Geometry check sheet. Reference: the model listing, model coordinates, mm. A direction names the side the tool comes from. Round coordinates to 2 decimals unless told otherwise and drop trailing zeros. Write each loop counter-clockwise with the first axis right and the second up, starting at its lowest first coordinate (ties: lowest second). Pieces come first, ordered by that corner, then holes.
Item 1: Cross-section at B-B (z = -0.2). State how many separate pieces and enclosed holes the cut face has, then the cut area to 3 significant figures.
Item 2: Cross-section at A-A (x = 70). Enter the section's corners in (y, z).
Item 3: Scan lines: probe 1 along Y at (x, z) = (0, -0.45); probe 2 along X at (y, z) = (0, -0.6); probe 3 along X at (y, z) = (-9.5, -0.05). Record each from-to range of solid material in increasing order.
Item 4: Depth check by flat-ended pin: P1, Ø3, axis at x = 77, y = -9.5, coming from the -Z side. Enter the tip coordinate at first touch or a pass-through.
Item 5: Access from +Z, -Z, +X, -X, +Y, -Y to the whole of each face (thin tool, end or side, straight path). Record for faces 1 (the face through (0, 7, -1.2)), 2 (the face through (79.1, -11.64, 0.02)), 3 (the face through (74, 0, 0)).
from build123d import *

# Parameters (mm, degrees)
SKETCH1_W                                            = 160
SKETCH1_H                                            = 25
BOSS_EXTRUDE1_DEPTH                                  = 1.5
SKETCH2_W                                            = 148
SKETCH2_H                                            = 13
CUT_EXTRUDE1_DEPTH                                   = 82.026230321
FILLET1_R                                            = 2
FILLET2_R                                            = 3
CSK_FOR_M2_SLOTTED_RAISED_CTSK_HEAD_SCRE_D           = 2.2
CSK_FOR_M2_SLOTTED_RAISED_CTSK_HEAD_SCRE_CSINK_D     = 4.5
CSK_FOR_M2_SLOTTED_RAISED_CTSK_HEAD_SCRE_CSINK_ANGLE = 90
MIRROR1_AT_THE_SECOND_PLANE_COPY_1_D                 = 2.2
MIRROR1_AT_THE_SECOND_PLANE_COPY_1_CSINK_D           = 4.5
MIRROR1_AT_THE_SECOND_PLANE_COPY_1_CSINK_ANGLE       = 90
SKETCH7_W                                            = 151
SKETCH7_H                                            = 16
CUT_EXTRUDE2_DEPTH                                   = 0.3
FILLET4_R                                            = 1


with BuildPart() as part:
    # Sketch1 → Boss-Extrude1 (new, symmetric)
    with BuildSketch(Plane.XY):
        Rectangle(SKETCH1_W, SKETCH1_H)
    extrude(amount=BOSS_EXTRUDE1_DEPTH, both=True)

    # Sketch2 → Cut-Extrude1 (cut, through all)
    with BuildSketch(Plane.XY.offset(1.5)):
        Rectangle(SKETCH2_W, SKETCH2_H)
    extrude(amount=-CUT_EXTRUDE1_DEPTH, mode=Mode.SUBTRACT)

    # Fillet1
    fillet1_edges = [part.edges().sort_by_distance(p)[0] for p in [
        (-74, -6.5, 0),
        (-74, 6.5, 0),
        (74, 6.5, 0),
        (74, -6.5, 0),
    ]]
    fillet(fillet1_edges, radius=FILLET1_R)

    # Fillet2
    fillet2_edges = [part.edges().sort_by_distance(p)[0] for p in [
        (80, -12.5, 0),
        (-80, -12.5, 0),
        (-80, 12.5, 0),
        (80, 12.5, 0),
    ]]
    fillet(fillet2_edges, radius=FILLET2_R)

    # CSK for M2 Slotted raised CTSK head screws1 (through all)
    with Locations(Plane(origin=(0, -9.5, 1.5), x_dir=(1, 0, 0), z_dir=(0, 0, 1))):
        with Locations((0, 0), (38.5, 0), (77, 0), (77, 9.5)):
            csk_for_m2_slotted_raised_ctsk_head_scre = CounterSinkHole(CSK_FOR_M2_SLOTTED_RAISED_CTSK_HEAD_SCRE_D / 2, CSK_FOR_M2_SLOTTED_RAISED_CTSK_HEAD_SCRE_CSINK_D / 2, counter_sink_angle=CSK_FOR_M2_SLOTTED_RAISED_CTSK_HEAD_SCRE_CSINK_ANGLE)

    # Mirror1: CSK for M2 Slotted raised CTSK head screws1 across plane
    add(csk_for_m2_slotted_raised_ctsk_head_scre.mirror(Plane.ZX), mode=Mode.SUBTRACT)

    # Mirror1 at the second plane: CSK for M2 Slotted raised CTSK head screws1 across plane
    add(csk_for_m2_slotted_raised_ctsk_head_scre.mirror(Plane(origin=(0, 0, 0), x_dir=(0, 0, 1), z_dir=(1, 0, 0))), mode=Mode.SUBTRACT)

    # Mirror1 at the second plane copy 1 (through all)
    with Locations(Plane(origin=(0, 9.5, 1.5), x_dir=(-1, 0, 0), z_dir=(0, 0, 1))):
        with Locations((0, 0), (38.5, 0), (77, 0), (77, 9.5)):
            CounterSinkHole(MIRROR1_AT_THE_SECOND_PLANE_COPY_1_D / 2, MIRROR1_AT_THE_SECOND_PLANE_COPY_1_CSINK_D / 2, counter_sink_angle=MIRROR1_AT_THE_SECOND_PLANE_COPY_1_CSINK_ANGLE)

    # Sketch7 → Cut-Extrude2 (cut)
    with BuildSketch(Plane(origin=(0, 0, -1.5), x_dir=(-1, 0, 0), z_dir=(0, 0, -1))):
        Rectangle(SKETCH7_W, SKETCH7_H)
    extrude(amount=-CUT_EXTRUDE2_DEPTH, mode=Mode.SUBTRACT)

    # Fillet4
    fillet4_edges = [part.edges().sort_by_distance(p)[0] for p in [
        (75.5, -8, -1.35),
        (75.5, 8, -1.35),
        (-75.5, 8, -1.35),
        (-75.5, -8, -1.35),
    ]]
    fillet(fillet4_edges, radius=FILLET4_R)


solid = part.part
Resolved:
1. separate pieces: 1
1. enclosed holes: 13
1. area: 2,030 mm2
2. outline: (-12.5, -1.5) - (-8, -1.5) - (-8, -1.2) - (-6.5, -1.2) - (-6.5, 1.5) - (-12.5, 1.5) - close; (6.5, -1.2) - (8, -1.2) - (8, -1.5) - (12.5, -1.5) - (12.5, 1.5) - (6.5, 1.5) - close
3. probe 1: y = -12.5 to -10.6, -8.4 to -6.5, 6.5 to 8.4, 10.6 to 12.5
3. probe 2: x = -80 to -78.1, -75.9 to -74, 74 to 75.9, 78.1 to 80
3. probe 3: x = -80 to -78.1, -75.9 to -39.6, -37.4 to -1.1, 1.1 to 37.4, 39.6 to 75.9, 78.1 to 80
4. P1: stops at z = -1.5
5. face 1: -Z
5. face 2: +Z, -Z, +X, -Y
5. face 3: +Z, -Z
